Work out the finished part from the listing and answer in its coordinate system (mm). Face numbers are marked on the shaded views. A direction names the side the tool comes from. Coordinates: 2 decimals unless noted, no trailing zeros. Loops run counter-clockwise (first coordinate to the right, second up) from the corner with the lowest first, then second, coordinate; pieces in that order, holes last. Notation, with made-up numbers: (21.5, 68) -> (48.5, 68) arc R14 ccw to (48.5, 87) -> close; hole circle Ø6 at (59.5, 7). An arc over 180 degrees is marked (long way). Use a Markdown table: item, result.
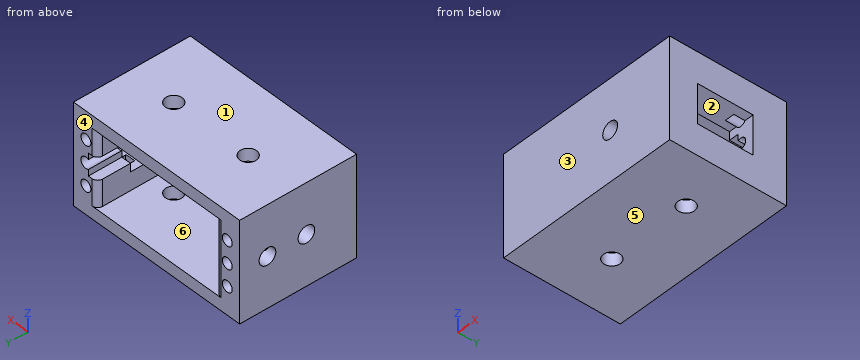
from build123d import *

# Parameters (mm, degrees)
CROQUIS1_W              = 33.5
CROQUIS1_H              = 18
SALIENTE_EXTRUIR1_DEPTH = 21
CROQUIS2_W              = 23.5
CROQUIS2_H              = 13.5
CORTAR_EXTRUIR1_DEPTH   = 16
CORTAR_EXTRUIR2_REACH   = 38.527
CROQUIS3_W              = 7
CROQUIS3_H              = 10
CROQUIS4_R              = 1
CORTAR_EXTRUIR3_DEPTH   = 8
CORTAR_EXTRUIR4_REACH   = 30.33
CROQUIS5_W              = 2
CROQUIS5_H              = 4
CORTAR_EXTRUIR5_REACH   = 26.851
CROQUIS6_R              = 1.5
CORTAR_EXTRUIR6_REACH   = 42.549
CROQUIS7_R              = 1.5
CROQUIS8_R              = 1.5
CORTAR_EXTRUIR7_DEPTH   = 33.335159
CORTAR_EXTRUIR8_REACH   = 30.33
CROQUIS9_W              = 0.25
CROQUIS9_H              = 13.5
REDONDEO1_R             = 1


with BuildPart() as part:
    # Croquis1 → Saliente-Extruir1 (new body)
    with BuildSketch(Plane(origin=(0, 0, 0), x_dir=(1, 0, 0), z_dir=(0, 1, 0))):
        Rectangle(CROQUIS1_W, CROQUIS1_H)
    extrude(amount=SALIENTE_EXTRUIR1_DEPTH)

    # Croquis2 → Cortar-Extruir1 (cut)
    with BuildSketch(Plane(origin=(0, 21, 0), x_dir=(1, 0, 0), z_dir=(0, 1, 0))):
        Rectangle(CROQUIS2_W, CROQUIS2_H)
    extrude(amount=-CORTAR_EXTRUIR1_DEPTH, mode=Mode.SUBTRACT)

    # Croquis3 → Cortar-Extruir2 (cut, up to next)
    with BuildSketch(Plane.ZY.offset(-11.75), mode=Mode.PRIVATE) as cortar_extruir2_sk1:
        with Locations((0, 10)):
            Rectangle(CROQUIS3_W, CROQUIS3_H)
    cortar_extruir2_tool1 = extrude(cortar_extruir2_sk1.sketch, amount=-CORTAR_EXTRUIR2_REACH, mode=Mode.PRIVATE) & part.part
    add(cortar_extruir2_tool1.solids().sort_by_distance((11.75, 10, 0))[0], mode=Mode.SUBTRACT)

    # Croquis4 → Cortar-Extruir3 (cut)
    with BuildSketch(Plane(origin=(0, 21, 0), x_dir=(1, 0, 0), z_dir=(0, 1, 0))):
        with Locations(Location((14.25, 0, 0), (0, 0, 270))):
            Circle(CROQUIS4_R)
        with Locations(Location((14.25, 4, 0), (0, 0, 270))):
            Circle(CROQUIS4_R)
        with Locations(Location((14.25, -4, 0), (0, 0, 30))):
            Circle(CROQUIS4_R)
        with Locations(Location((-14.25, -4, 0), (0, 0, 270))):
            Circle(CROQUIS4_R)
        with Locations(Location((-14.25, 0, 0), (0, 0, 90))):
            Circle(CROQUIS4_R)
        with Locations(Location((-14.25, 4, 0), (0, 0, 90))):
            Circle(CROQUIS4_R)
    extrude(amount=-CORTAR_EXTRUIR3_DEPTH, mode=Mode.SUBTRACT)

    # Croquis5 → Cortar-Extruir4 (cut, up to next)
    with BuildSketch(Plane(origin=(0, 21, 0), x_dir=(1, 0, 0), z_dir=(0, 1, 0)), mode=Mode.PRIVATE) as cortar_extruir4_sk1:
        with Locations((12.75, 0)):
            Rectangle(CROQUIS5_W, CROQUIS5_H)
    cortar_extruir4_tool1 = extrude(cortar_extruir4_sk1.sketch, amount=-CORTAR_EXTRUIR4_REACH, mode=Mode.PRIVATE) & part.part
    add(cortar_extruir4_tool1.solids().sort_by_distance((12.75, 21, 0))[0], mode=Mode.SUBTRACT)

    # Croquis6 → Cortar-Extruir5 (cut, up to next)
    with BuildSketch(Plane(origin=(0, 5, 0), x_dir=(1, 0, 0), z_dir=(0, 1, 0)), mode=Mode.PRIVATE) as cortar_extruir5_sk1:
        with Locations(Location((4.75, 0, 0), (0, 0, 270))):
            Circle(CROQUIS6_R)
    cortar_extruir5_tool1 = extrude(cortar_extruir5_sk1.sketch, amount=-CORTAR_EXTRUIR5_REACH, mode=Mode.PRIVATE) & part.part
    add(cortar_extruir5_tool1.solids().sort_by_distance((4.75, 5, 0))[0], mode=Mode.SUBTRACT)

    # Croquis7 → Cortar-Extruir6 (cut, up to next)
    with BuildSketch(Plane.ZY.offset(16.75), mode=Mode.PRIVATE) as cortar_extruir6_sk1:
        with Locations((0, 16)):
            Circle(CROQUIS7_R)
    cortar_extruir6_tool1 = extrude(cortar_extruir6_sk1.sketch, amount=-CORTAR_EXTRUIR6_REACH, mode=Mode.PRIVATE) & part.part
    # Croquis7 → Cortar-Extruir6 (cut, up to next)
    with BuildSketch(Plane.ZY.offset(16.75), mode=Mode.PRIVATE) as cortar_extruir6_sk2:
        with Locations((0, 9)):
            Circle(CROQUIS7_R)
    cortar_extruir6_tool2 = extrude(cortar_extruir6_sk2.sketch, amount=-CORTAR_EXTRUIR6_REACH, mode=Mode.PRIVATE) & part.part
    add(cortar_extruir6_tool1.solids().sort_by_distance((-16.75, 16, 0))[0], mode=Mode.SUBTRACT)
    add(cortar_extruir6_tool2.solids().sort_by_distance((-16.75, 9, 0))[0], mode=Mode.SUBTRACT)

    # Croquis8 → Cortar-Extruir7 (cut, through all)
    with BuildSketch(Plane(origin=(0, 0, -9), x_dir=(-1, 0, 0), z_dir=(0, 0, -1))):
        with Locations((-7.75, 11)):
            Circle(CROQUIS8_R)
        with Locations((7.25, 11)):
            Circle(CROQUIS8_R)
    extrude(amount=-CORTAR_EXTRUIR7_DEPTH, mode=Mode.SUBTRACT)

    # Cortar-Extruir8: up to this face of the body (flat: up to its plane)
    cortar_extruir8_end = Plane(part.part.faces().sort_by_distance((1.347622457, 5, 0))[0])
    # Croquis9 → Cortar-Extruir8 (cut, up to the picked face)
    with BuildSketch(Plane(origin=(0, 21, 0), x_dir=(1, 0, 0), z_dir=(0, 1, 0)), mode=Mode.PRIVATE) as cortar_extruir8_sk1:
        with Locations((-11.875, 0)):
            Rectangle(CROQUIS9_W, CROQUIS9_H)
    cortar_extruir8_tool1 = split(extrude(cortar_extruir8_sk1.sketch, amount=-CORTAR_EXTRUIR8_REACH, mode=Mode.PRIVATE), bisect_by=cortar_extruir8_end, keep=Keep.BOTH, mode=Mode.PRIVATE)
    # Croquis9 → Cortar-Extruir8 (cut, up to the picked face)
    with BuildSketch(Plane(origin=(0, 21, 0), x_dir=(1, 0, 0), z_dir=(0, 1, 0)), mode=Mode.PRIVATE) as cortar_extruir8_sk2:
        with Locations((11.875, 0)):
            Rectangle(CROQUIS9_W, CROQUIS9_H)
    cortar_extruir8_tool2 = split(extrude(cortar_extruir8_sk2.sketch, amount=-CORTAR_EXTRUIR8_REACH, mode=Mode.PRIVATE), bisect_by=cortar_extruir8_end, keep=Keep.BOTH, mode=Mode.PRIVATE)
    add(cortar_extruir8_tool1.solids().sort_by(Axis((-11.875, 21, 0), (0, -1, 0)))[0], mode=Mode.SUBTRACT)
    add(cortar_extruir8_tool2.solids().sort_by(Axis((11.875, 21, 0), (0, -1, 0)))[0], mode=Mode.SUBTRACT)

    # Redondeo1
    redondeo1_edges = [part.edges().sort_by_distance(p)[0] for p in [
        (-12, 21, 0),
        (12, 21, -4.375),
        (12, 21, 4.375),
    ]]
    fillet(redondeo1_edges, radius=REDONDEO1_R)


solid = part.part
Q1. For the marked faces 5 and 6, determine the directions among +Z, -Z, +X, -X, +Y, -Y from which every point of the face is accessible in a straight line to the end or side of a thin tool.
Solved:
| item | result |
|---|---|
| face 5 | -Z, +X, -X, +Y, -Y |
| face 6 | +Y |
Q2. Section A-A on x = -7.25 is taken. Determine the outline of the cut face in (y, z), and give its area (4 significant figures).
Solved:
| item | result |
|---|---|
| outline | (0, -9) -> (9.5, -9) -> (9.5, -6.75) -> (5, -6.75) -> (5, 6.75) -> (9.5, 6.75) -> (9.5, 9) -> (0, 9) -> close; (12.5, -9) -> (21, -9) -> (21, -6.75) -> (12.5, -6.75) -> close; (12.5, 6.75) -> (21, 6.75) -> (21, 9) -> (12.5, 9) -> close |
| area | 148.5 mm² |
Q3. Section D-D on x = -3.5 is taken. Determine the outline of the cut face in (y, z).
Solved:
| item | result |
|---|---|
| outline | (0, -9) -> (21, -9) -> (21, -6.75) -> (5, -6.75) -> (5, 6.75) -> (21, 6.75) -> (21, 9) -> (0, 9) -> close |
Q4. Given pin 1 Ø1.8 at (x, z) = (14.25, -4) entering from +Y; pin 2 Ø3.5 at (y, z) = (9, 0) entering from +X, each flat-ended and moving along its own axis, determine where each tip first touches the part or whether it passes through.
Solved:
| item | result |
|---|---|
| pin 1 | y = 13 |
| pin 2 | x = -12 |
Q5. Section C-C on z = 4 is taken. Determine the outline of the cut face in (x, y), and give its area (3 significant figures).
Solved:
| item | result |
|---|---|
| outline | (-16.75, 0) -> (16.75, 0) -> (16.75, 21) -> (15.25, 21) -> (15.25, 13) -> (13.25, 13) -> (13.25, 21) -> (13, 21) arc R1 ccw to (12, 20) -> (12, 5) -> (-12, 5) -> (-12, 20) arc R1 ccw to (-13, 21) -> (-13.25, 21) -> (-13.25, 13) -> (-15.25, 13) -> (-15.25, 21) -> (-16.75, 21) -> close |
| area | 287 mm² |
Q6. Consider line 1 (X direction, y = 19.2, z = 0); line 2 (X direction, y = 18.25, z = 4); line 3 (Y direction, x = -13, z = -1). Determine where each line is inside the solid, lowest interval first. Write a range as [from, to].
Solved:
| item | result |
|---|---|
| line 1 | [-16.75, -15.25], [-13.25, -12], [15.25, 16.75] |
| line 2 | [-16.75, -15.25], [-13.25, -12], [12, 13.25], [15.25, 16.75] |
| line 3 | [0, 7.88], [10.12, 14.88], [17.12, 21] |
Q7. Determine the mould class of the marked faces 1, 2, 3 and 4 for opening direction Y: pulls with the +Y half, pulls with the -Y half, needs draft (parallel to the pull), parting line crosses it, or undercut.
Solved:
| item | result |
|---|---|
| face 1 | needs draft |
| face 2 | undercut |
| face 3 | pulls with the -Y half |
| face 4 | pulls with the +Y half |
Q8. Section B-B on y = 9 is taken. Determine the outline of the cut face in (x, z).
Solved:
| item | result |
|---|---|
| outline | (-16.75, -9) -> (16.75, -9) -> (16.75, -3.5) -> (12, -3.5) -> (12, -6.75) -> (-12, -6.75) -> (-12, -1.5) -> (-16.75, -1.5) -> close; (-16.75, 1.5) -> (-12, 1.5) -> (-12, 6.75) -> (12, 6.75) -> (12, 3.5) -> (16.75, 3.5) -> (16.75, 9) -> (-16.75, 9) -> close |
